Geometry check sheet. Reference: the model listing, model coordinates, mm. A direction names the side the tool comes from. Coordinates: 2 decimals unless noted, no trailing zeros. Write each loop counter-clockwise with the first axis right and the second up, starting at its lowest first coordinate (ties: lowest second). Pieces come first, ordered by that corner, then holes. Notation, with made-up numbers: (34.5, 14.5) -> (46.5, 14.5) arc R31 ccw to (46.5, 50.5) -> close; hole circle Ø8 at (15.5, -32). An arc over 180 degrees is marked (long way). Answer as CSV lines item,"result".
```python
from build123d import *

# Parameters (mm, degrees)
F0_R     = 13.49375
F1_DEPTH = 45
F2_W     = 5
F2_H     = 35
F3_DEPTH = 33.8074


with BuildPart() as f1:
    # F0 (on Top) → F1 (new body)
    with BuildSketch(Plane.XY):
        with BuildLine():
            Line((14.050669, 12.700597), (-17.699331, 12.700597))
            Line((-17.699331, 12.700597), (-17.699331, -9.235959))
            ThreePointArc((-17.699331, -9.235959), (-2.403239, -26.220174), (14.050669, -10.355026))
            Line((14.050669, -10.355026), (14.050669, -10.316926))
            Line((14.050669, -10.316926), (14.050669, 12.700597))
        make_face()
        with Locations((-1.843381, -10.335976)):
            Circle(F0_R, mode=Mode.SUBTRACT)
    extrude(amount=F1_DEPTH)

    # F2 (on face) → F3 (cut)
    with BuildSketch(Plane.YZ.offset(14.050669)):
        with Locations((7.700597, 22.5)):
            Rectangle(F2_W, F2_H)
    extrude(amount=-F3_DEPTH, mode=Mode.SUBTRACT)


solid = f1.part
```
Item 1: Release check for a two-part mould opening along Z. For faces 1 (the flat face through (-2, 6, 45)), 2 (the flat face through (-2, 5.201, 22)), 3 (the cylindrical face through (-2.8, -26.2, 22.2)) record: +Z half, -Z half, draft (parallel to the pull), parting line (faces both ways), or undercut.
Responses:
face 1,"+Z half"
face 2,"undercut"
face 3,"draft"
Item 2: Set-up check for faces 4 (the flat face through (14.051, -2, 22)), 5 (the flat face through (-2, 10.201, 22)): record each of +Z, -Z, +X, -X, +Y, -Y from which the full face is reachable in a straight line by a thin tool's end or side.
Responses:
face 4,"+Z, -Z, +X, +Y, -Y"
face 5,"+X, -X"
Item 3: Cross-section at A-A, the plane y = 8.5. Record the cut outline in (x, z), plus the area to 4 significant figures.
Responses:
outline,"(-17.7, 0) -> (14.05, 0) -> (14.05, 5) -> (-17.7, 5) -> close; (-17.7, 40) -> (14.05, 40) -> (14.05, 45) -> (-17.7, 45) -> close"
area,"317.5 mm2"
Item 4: Cross-section at B-B, the plane x = 5. Record the cut outline in (y, z).
Responses:
outline,"(-24.68, 0) -> (-21.97, 0) -> (-21.97, 45) -> (-24.68, 45) -> close; (1.29, 0) -> (12.7, 0) -> (12.7, 45) -> (1.29, 45) -> close; hole (5.2, 5) -> (10.2, 5) -> (10.2, 40) -> (5.2, 40) -> close"
Item 5: Thickness scan on probe 1 along Y at (x, z) = (-1.5, 8.5); probe 2 along Y at (x, z) = (-14, 32.5) (3 decimals); probe 3 along X at (y, z) = (-10, 42). Record the ranges inside material, lowest first.
Responses:
probe 1,"y = -26.23 to -23.83, 3.15 to 5.2, 10.2 to 12.7"
probe 2,"y = -20.575 to -16.192, -4.48 to 5.201, 10.201 to 12.701"
probe 3,"x = -17.73 to -15.33, 11.65 to 14.05"
Item 6: Cross-section at D-D, the plane x = -12.5. Record the cut outline in (y, z).
Responses:
outline,"(-22.13, 0) -> (-18.61, 0) -> (-18.61, 45) -> (-22.13, 45) -> close; (-2.06, 0) -> (12.7, 0) -> (12.7, 45) -> (-2.06, 45) -> close; hole (5.2, 5) -> (10.2, 5) -> (10.2, 40) -> (5.2, 40) -> close"
Item 7: Depth check by flat-ended pin: pin 1 Ø8 at (x, z) = (8, 8.5) entering from -Y; pin 2 Ø8 at (y, z) = (-21.5, 23.5) entering from +X; pin 3 Ø4 at (x, z) = (-10, 34) entering from -Y. Enter the tip coordinate at first touch or a pass-through.
Responses:
pin 1,"stops at y = -25.12"
pin 2,"stops at x = 12.34"
pin 3,"stops at y = -24.99"
